Here's how the part is built. I have some questions about the finished solid (model axes, mm). A direction names the side the tool comes from. Round coordinates to 2 decimals unless told otherwise and drop trailing zeros. Loops run counter-clockwise (first coordinate to the right, second up) from the corner with the lowest first, then second, coordinate; pieces in that order, holes last. Notation, with made-up numbers: M 7.25,22.5 L 12.25,22.5 A13 ccw 12.25,40.5 Z; hole C -14,30 d11. An arc over 180 degrees is marked long. Answer as a JSON object with one key per item and string values.
from build123d import *

# Parameters (mm, degrees)
F0_W     = 4
F0_H     = 78
F1_DEPTH = 9.17
F2_R     = 48
F2_R_2   = 44.915
F3_DEPTH = 3
F4_R     = 52
F4_R_2   = 45.823457
F5_DEPTH = 1
F6_W     = 70
F6_H     = 60
F7_DEPTH = 3


with BuildPart() as f1:
    # F0 (on Front) → F1 (new body)
    with BuildSketch(Plane.XZ):
        Polygon((56.75, 39), (56.75, 57), (-56.75, 57), (-56.75, -57), (56.75, -57), (56.75, -39), align=None)
        with Locations((58.75, 0)):
            Rectangle(F0_W, F0_H)
    extrude(amount=F1_DEPTH)

    # F2 (on face) → F3 (join)
    with BuildSketch(Plane.XZ.offset(9.17)):
        Circle(F2_R)
        Circle(F2_R_2, mode=Mode.SUBTRACT)
    extrude(amount=F3_DEPTH)

    # F4 (on face) → F5 (join)
    with BuildSketch(Plane.XZ.offset(9.17)):
        Circle(F4_R)
        Circle(F4_R_2, mode=Mode.SUBTRACT)
    extrude(amount=F5_DEPTH)

    # F6 (on face) → F7 (cut)
    with BuildSketch(Plane.XZ.offset(9.17)):
        Rectangle(F6_W, F6_H)
    extrude(amount=-F7_DEPTH, mode=Mode.SUBTRACT)


solid = f1.part
Item 1: If I drill on L1, parallel to Z at x = 0, y = -10.4 (3 decimals); L2, parallel to Z at x = 15, y = -8.5, over which ranges is the centre line in solid material (lowest first)? Write a range as from..to.
Solution:
{"L1": "z = -48..-44.915, 44.915..48", "L2": "z = -57..-30, 30..57"}
Item 2: I want a section at B-B on z = 0. List the corners of the cut face in (x, y) for me (3 decimals).
Solution:
{"outline": "M -56.75,-9.17 L -52,-9.17 L -52,-10.17 L -48,-10.17 L -48,-12.17 L -44.915,-12.17 L -44.915,-9.17 L -35,-9.17 L -35,-6.17 L 35,-6.17 L 35,-9.17 L 44.915,-9.17 L 44.915,-12.17 L 48,-12.17 L 48,-10.17 L 52,-10.17 L 52,-9.17 L 60.75,-9.17 L 60.75,0 L -56.75,0 Z"}
Item 3: I want a section at D-D on x = 43.5. List the corners of the cut face in (y, z) for me, plus the area to 3 significant figures.
Solution:
{"outline": "M -12.17,-20.29 L -10.17,-20.29 L -10.17,-28.49 L -9.17,-28.49 L -9.17,-57 L 0,-57 L 0,57 L -9.17,57 L -9.17,28.49 L -10.17,28.49 L -10.17,20.29 L -12.17,20.29 L -12.17,11.19 L -9.17,11.19 L -9.17,-11.19 L -12.17,-11.19 Z", "area": "1,120 mm2"}
Item 4: I want a section at A-A on x = 0. List the corners of the cut face in (y, z) for me (3 decimals).
Solution:
{"outline": "M -12.17,-48 L -10.17,-48 L -10.17,-52 L -9.17,-52 L -9.17,-57 L 0,-57 L 0,57 L -9.17,57 L -9.17,52 L -10.17,52 L -10.17,48 L -12.17,48 L -12.17,44.915 L -9.17,44.915 L -9.17,30 L -6.17,30 L -6.17,-30 L -9.17,-30 L -9.17,-44.915 L -12.17,-44.915 Z"}
Item 5: For P1, Ø1.5, axis at x = -34.5, z = 26.5, coming from the -Y side; P2, Ø1.5, axis at x = 31, z = 28, coming from the -Y side; P3, Ø4.5, axis at y = -5, z = -49, coming from the +X side, each with a flat end and sliding along its axis, tell me the tip position at first contact or that it passes through.
Solution:
{"P1": "stops at y = -9.17", "P2": "stops at y = -6.17", "P3": "stops at x = 56.75"}
Item 6: I want a section at C-C on z = 36.5. List the corners of the cut face in (x, y) for me.
Solution:
{"outline": "M -56.75,-9.17 L -37.04,-9.17 L -37.04,-10.17 L -31.17,-10.17 L -31.17,-12.17 L -26.17,-12.17 L -26.17,-9.17 L 26.17,-9.17 L 26.17,-12.17 L 31.17,-12.17 L 31.17,-10.17 L 37.04,-10.17 L 37.04,-9.17 L 60.75,-9.17 L 60.75,0 L -56.75,0 Z"}
Item 7: For faces 1 (the face through (14, -9.17, 51)), 2 (the face through (32, -12.17, -32)), 3 (the face through (59, -5, -39)), which set-ups out of +Z, -Z, +X, -X, +Y, -Y let a thin tool reach every point of the face, with its end or its side?
Solution:
{"face 1": "-Y", "face 2": "+Z, -Z, +X, -X, -Y", "face 3": "-Z, +X, +Y, -Y"}
